from build123d import *

# Parameters (mm, degrees)
BOSS_EXTRUDE1_DEPTH = 5
SKETCH2_W           = 5
SKETCH2_H           = 90
CUT_EXTRUDE1_DEPTH  = 79.262379212
BOSS_EXTRUDE3_DEPTH = 60
BOSS_EXTRUDE4_DEPTH = 4
SKETCH5_W           = 90
SKETCH5_H           = 80
CUT_EXTRUDE2_DEPTH  = 4


with BuildPart() as part:
    # Sketch1 → Boss-Extrude1 (new body)
    with BuildSketch(Plane(origin=(0, 0, 0), x_dir=(1, 0, 0), z_dir=(0, 1, 0))):
        with BuildLine():
            Line((-40, 60), (40, 60))
            ThreePointArc((40, 60), (47.071067812, 57.071067812), (50, 50))
            Line((50, 50), (50, -50))
            ThreePointArc((50, -50), (47.071067812, -57.071067812), (40, -60))
            Line((40, -60), (-40, -60))
            ThreePointArc((-40, -60), (-47.071067812, -57.071067812), (-50, -50))
            Line((-50, -50), (-50, 50))
            ThreePointArc((-50, 50), (-47.071067812, 57.071067812), (-40, 60))
        make_face()
    extrude(amount=BOSS_EXTRUDE1_DEPTH)

    # Sketch2 → Cut-Extrude1 (cut, through all)
    with BuildSketch(Plane(origin=(0, 5, 0), x_dir=(1, 0, 0), z_dir=(0, 1, 0))):
        with Locations((-42.5, 0)):
            Rectangle(SKETCH2_W, SKETCH2_H)
        with Locations((42.5, 0)):
            Rectangle(SKETCH2_W, SKETCH2_H)
    extrude(amount=-CUT_EXTRUDE1_DEPTH, mode=Mode.SUBTRACT)

    # Sketch3 → Boss-Extrude3 (add)
    with BuildSketch(Plane(origin=(0, 5, 0), x_dir=(1, 0, 0), z_dir=(0, 1, 0))):
        with BuildLine():
            Line((-50, 50), (-40, 50))
            Line((-40, 50), (-40, 60))
            ThreePointArc((-40, 60), (-47.071067812, 57.071067812), (-50, 50))
        make_face()
        with BuildLine():
            Line((40, 60), (40, 50))
            Line((40, 50), (50, 50))
            ThreePointArc((50, 50), (47.071067812, 57.071067812), (40, 60))
        make_face()
        with BuildLine():
            Line((-50, -50), (-40, -50))
            Line((-40, -50), (-40, -60))
            ThreePointArc((-40, -60), (-47.071067812, -57.071067812), (-50, -50))
        make_face()
        with BuildLine():
            Line((50, -50), (40, -50))
            Line((40, -50), (40, -60))
            ThreePointArc((40, -60), (47.071067812, -57.071067812), (50, -50))
        make_face()
    extrude(amount=BOSS_EXTRUDE3_DEPTH)

    # Sketch4 → Boss-Extrude4 (add)
    with BuildSketch(Plane(origin=(0, 65, 0), x_dir=(1, 0, 0), z_dir=(0, 1, 0))):
        with BuildLine():
            Line((50, -50), (50, 50))
            ThreePointArc((50, 50), (47.071067812, 57.071067812), (40, 60))
            Line((40, 60), (-40, 60))
            ThreePointArc((-40, 60), (-47.071067812, 57.071067812), (-50, 50))
            Line((-50, 50), (-50, -50))
            ThreePointArc((-50, -50), (-47.071067812, -57.071067812), (-40, -60))
            Line((-40, -60), (40, -60))
            ThreePointArc((40, -60), (47.071067812, -57.071067812), (50, -50))
        make_face()
    extrude(amount=BOSS_EXTRUDE4_DEPTH)

    # Sketch5 → Cut-Extrude2 (cut)
    with BuildSketch(Plane(origin=(0, 69, 0), x_dir=(1, 0, 0), z_dir=(0, 1, 0))):
        with Locations((0, -15)):
            Rectangle(SKETCH5_W, SKETCH5_H)
    extrude(amount=-CUT_EXTRUDE2_DEPTH, mode=Mode.SUBTRACT)


solid = part.part
Geometry check sheet. Reference: the model listing, model coordinates, mm. A direction names the side the tool comes from. Round coordinates to 2 decimals unless told otherwise and drop trailing zeros. Order: outer loops, then holes, each group sorted by start corner. A loop starts at its lowest first (then second) coordinate and runs counter-clockwise, first axis right, second up. Notation, with made-up numbers: M -4,11.5 L 10,11.5 A14 ccw 10,23.5 Z; hole C 5.5,18 d1. An arc over 180 degrees is marked long. Answer in a Markdown table with one row per item. Add a question column.
Item 1: Draft check along X on faces 4 (the face through (42, 3, -45)), 5 (the face through (1, 0, -1)), 6 (the face through (-45, 67, 16)), 7 (the face through (50, 67, 1)). Enter one of: released by +X, released by -X, zero draft, split by the parting line, or undercut.
Item 2: Set-up check for faces 1 (the face through (45, 35, 50)), 2 (the face through (-43, 3, 45)), 3 (the face through (-1, 67, -25)): record each of +Z, -Z, +X, -X, +Y, -Y from which the full face is reachable in a straight line by a thin tool's end or side.
Item 3: Depth check by flat-ended pin: pin 1 Ø3 at (x, z) = (-13.5, 22.5) entering from -Y; pin 2 Ø3 at (x, y) = (43.5, 24) entering from +Z; pin 3 Ø1.5 at (x, y) = (41.5, 2.5) entering from -Z; pin 4 Ø5 at (x, z) = (-5.5, -21.5) entering from +Y. Enter the tip coordinate at first touch or a pass-through.
Item 4: Sectioned sample at C-C, the plane x = -7. Enter the section's corners in (y, z).
Item 5: Sectioned sample at B-B, the plane z = -15. Enter the section's corners in (x, y).
Item 6: Material ranges on L1, parallel to Y at x = -37, z = -52; L2, parallel to Y at x = -3, z = -13.5; L3, parallel to Z at x = -42, y = 10.5, recorded low to high. Write a range as [from, to].
Item 7: Sectioned sample at A-A, the plane y = 43. Enter the section's corners in (x, z).
Filled in:
| question | item | result |
|---|---|---|
| 1 | face 4 | undercut |
| 1 | face 5 | zero draft |
| 1 | face 6 | undercut |
| 1 | face 7 | released by +X |
| 2 | face 1 | +X, -X |
| 2 | face 2 | +Y, -Y |
| 2 | face 3 | +Y |
| 3 | pin 1 | stops at y = 0 |
| 3 | pin 2 | stops at z = 59.8 |
| 3 | pin 3 | stops at z = -59.97 |
| 3 | pin 4 | stops at y = 5 |
| 4 | outline | M 0,-60 L 5,-60 L 5,60 L 0,60 Z; M 65,-60 L 69,-60 L 69,-25 L 65,-25 Z; M 65,55 L 69,55 L 69,60 L 65,60 Z |
| 5 | outline | M -50,0 L -45,0 L -45,5 L -50,5 Z; M -50,65 L -45,65 L -45,69 L -50,69 Z; M -40,0 L 40,0 L 40,5 L -40,5 Z; M 45,0 L 50,0 L 50,5 L 45,5 Z; M 45,65 L 50,65 L 50,69 L 45,69 Z |
| 6 | L1 | y = [0, 5], [65, 69] |
| 6 | L2 | y = [0, 5] |
| 6 | L3 | z = [-59.8, -50], [50, 59.8] |
| 7 | outline | M -50,-50 A10 ccw -40,-60 L -40,-50 Z; M -50,50 L -40,50 L -40,60 A10 ccw Z; M 40,-60 A10 ccw 50,-50 L 40,-50 Z; M 40,50 L 50,50 A10 ccw 40,60 Z |
